```python
from build123d import *

# Parameters (mm, degrees)
SKETCH1_W           = 6.35
SKETCH1_H           = 19.05
SKETCH1_H_2         = 4.572
BOSS_EXTRUDE1_DEPTH = 4.572


with BuildPart() as part:
    # Sketch1 → Boss-Extrude1 (new body)
    with BuildSketch(Plane.XY):
        Polygon((19.05, -5.08), (29.845, -5.08), (29.845, 0), (6.35, 0), (0, 0), (0, -5.08), (12.7, -5.08), align=None)
        with Locations((3.175, 9.525)):
            Rectangle(SKETCH1_W, SKETCH1_H)
        with Locations((15.875, -7.366)):
            Rectangle(SKETCH1_W, SKETCH1_H_2)
        Polygon((29.845, 0), (29.845, -5.08), (38.1, -5.08), (44.45, -5.08), (59.69, -5.08), (59.69, 0), (53.34, 0), align=None)
        with Locations((56.515, 9.525)):
            Rectangle(SKETCH1_W, SKETCH1_H)
        with Locations((41.275, -7.366)):
            Rectangle(SKETCH1_W, SKETCH1_H_2)
    extrude(amount=BOSS_EXTRUDE1_DEPTH)


solid = part.part
```
Design review of the part built by this model. Coordinates are the model's own, in mm. A direction names the side the tool comes from. Give positions to 0.01 mm unless a question says otherwise; leave off trailing zeros. Write each loop counter-clockwise with the first axis right and the second up, starting at its lowest first coordinate (ties: lowest second). Pieces come first, ordered by that corner, then holes.
(1) Add section D-D (x = 41). Give the boundary of the cut face in (y, z), and give its area (3 significant figures).
Checked values:
outline: (-9.65, 0) - (0, 0) - (0, 4.57) - (-9.65, 4.57) - close
area: 44.1 mm2
(2) Mouldability with a two-part tool opening along X and no side actions: class faces 6 (the face through (44.45, -7, 2)), 7 (the face through (0, 7, 2)), 8 (the face through (19.05, -7, 2)), 9 (the face through (29, -1, 0)) as +X half, -X half, draft (parallel to the pull), parting line (faces both ways), or undercut.
Checked values:
face 6: +X half
face 7: -X half
face 8: undercut
face 9: draft
(3) Add section C-C (x = 32.5). Give the boundary of the cut face in (y, z).
Checked values:
outline: (-5.08, 0) - (0, 0) - (0, 4.57) - (-5.08, 4.57) - close
(4) Clearance check with flat-ended pins moving along their axes: pin 1 Ø1.4 at (x, z) = (5, 3) entering from -Y; pin 2 Ø1.4 at (x, z) = (25, 3) entering from +Y. State where each tip first meets the part, or that it passes through.
Checked values:
pin 1: stops at y = -5.08
pin 2: stops at y = 0
(5) Wall thickness on line 1 along X through (y, z) = (4, 3.9); line 2 along X through (y, z) = (-6.25, 1.25); line 3 along Y through (x, z) = (56, 3.15): over which ranges is each line inside the solid? List them lowest first.
Checked values:
line 1: x = 0 to 6.35, 53.34 to 59.69
line 2: x = 12.7 to 19.05, 38.1 to 44.45
line 3: y = -5.08 to 19.05
(6) Add section A-A (y = 2.75). Give the boundary of the cut face in (x, z).
Checked values:
outline: (0, 0) - (6.35, 0) - (6.35, 4.57) - (0, 4.57) - close; (53.34, 0) - (59.69, 0) - (59.69, 4.57) - (53.34, 4.57) - close
(7) Add section B-B (z = 0.65). Give the boundary of the cut face in (x, y), and give its area (3 significant figures).
Checked values:
outline: (0, -5.08) - (12.7, -5.08) - (12.7, -9.65) - (19.05, -9.65) - (19.05, -5.08) - (38.1, -5.08) - (38.1, -9.65) - (44.45, -9.65) - (44.45, -5.08) - (59.69, -5.08) - (59.69, 19.05) - (53.34, 19.05) - (53.34, 0) - (6.35, 0) - (6.35, 19.05) - (0, 19.05) - close
area: 603 mm2
(8) Tool access review of faces 1 (the face through (52, -5.08, 2)), 2 (the face through (6, -5.08, 2)), 3 (the face through (28, -5.08, 2)), 4 (the face through (29, -1, 4.572)), 5 (the face through (30, 0, 2)): name each direction out of +Z, -Z, +X, -X, +Y, -Y from which nothing blocks a thin tool from reaching the whole face with its end or side.
Checked values:
face 1: +Z, -Z, +X, -Y
face 2: +Z, -Z, -X, -Y
face 3: +Z, -Z, -Y
face 4: +Z, +X, -X, +Y, -Y
face 5: +Z, -Z, +Y
